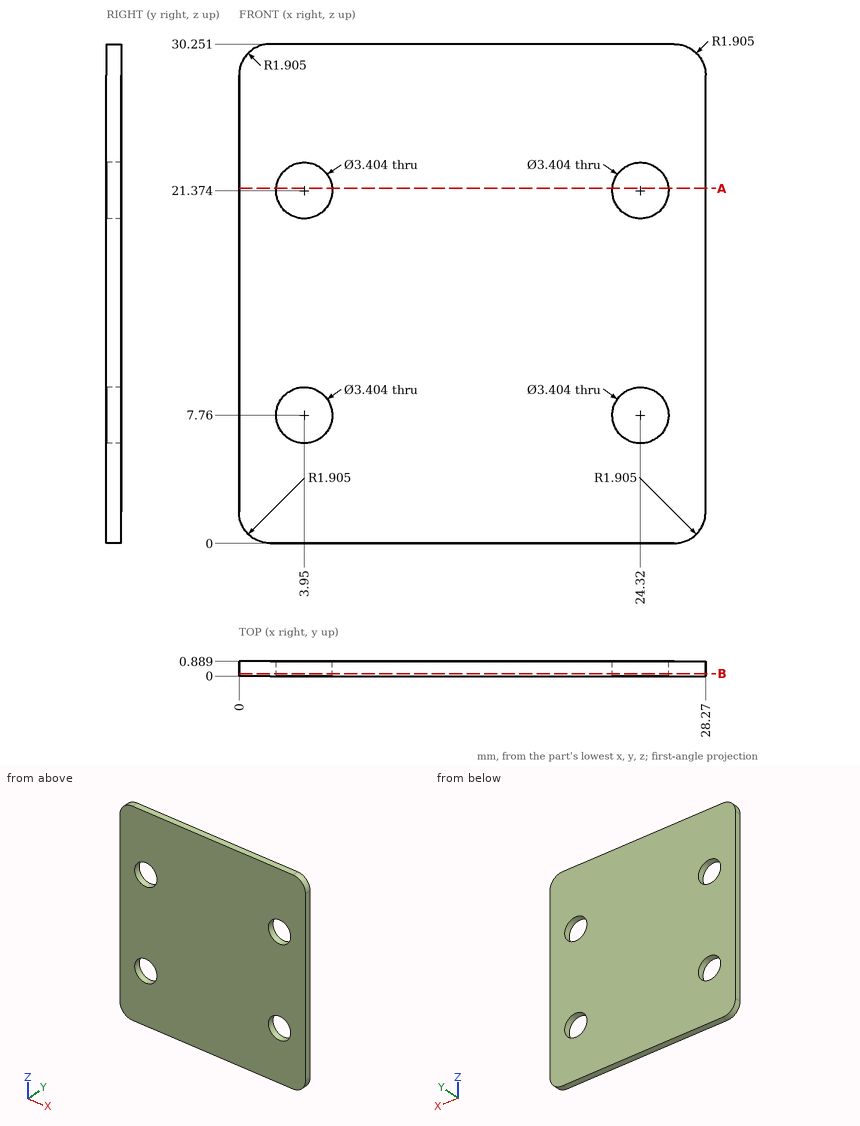
Here's the drawing with two shaded views (mm, measured from the low corner). I have some questions. Coordinates: 2 decimals unless noted, no trailing zeros. Loops run counter-clockwise (first coordinate to the right, second up) from the corner with the lowest first, then second, coordinate; pieces in that order, holes last. Notation, with made-up numbers: M 5.25,61 L 25.25,61 A17 ccw 25.25,74 Z; hole C 45,24 d2. An arc over 180 degrees is marked long. Return JSON: item names as keys, results as strings. Group by question number.
Item 1: Imagine slicing it at B-B (y = 0.15). Give the number of separate pieces and of enclosed holes in the cut face, and give its area (3 significant figures).
Item 2: If I drill on L1, parallel to X at y = 0.8, z = 22.5 (1 decimal); L2, parallel to Z at x = 1.5, y = 0.4 (1 decimal), over which ranges is the centre line in solid material (lowest first)? Write a range as from..to.
Item 3: I'm going to push a flat-ended pin straight in: pin 1 Ø3 at (x, z) = (24.32, 21.37) entering from +Y. Where does the tip first touch, or does it pass through?
Item 4: Imagine slicing it at A-A (z = 21.5). Please give me the cut outline in (x, y).
Verdict:
{
 "1": {"separate pieces": "1", "enclosed holes": "4", "area": "816 mm^2"},
 "2": {"L1": "x = 0..2.7, 5.2..23, 25.6..28.3", "L2": "z = 0..30.2"},
 "3": {"pin 1": "passes through"},
 "4": {"outline": "M 0,0 L 2.25,0 L 2.25,0.89 L 0,0.89 Z; M 5.65,0 L 22.62,0 L 22.62,0.89 L 5.65,0.89 Z; M 26.02,0 L 28.27,0 L 28.27,0.89 L 26.02,0.89 Z"}
}
